from build123d import *

# Parameters (mm, degrees)
CROQUIS1_W              = 200
CROQUIS1_H              = 150
SALIENTE_EXTRUIR1_DEPTH = 3
CROQUIS2_W              = 3
CROQUIS2_H              = 150
SALIENTE_EXTRUIR2_DEPTH = 134
CROQUIS3_W              = 200
CROQUIS3_H              = 150
SALIENTE_EXTRUIR3_DEPTH = 3


with BuildPart() as part:
    # Croquis1 → Saliente-Extruir1 (new body)
    with BuildSketch(Plane(origin=(0, 0, 0), x_dir=(1, 0, 0), z_dir=(0, 1, 0))):
        with Locations((100, 75)):
            Rectangle(CROQUIS1_W, CROQUIS1_H)
    extrude(amount=SALIENTE_EXTRUIR1_DEPTH)

    # Croquis2 → Saliente-Extruir2 (add)
    with BuildSketch(Plane(origin=(0, 3, 0), x_dir=(1, 0, 0), z_dir=(0, 1, 0))):
        with Locations((1.5, 75)):
            Rectangle(CROQUIS2_W, CROQUIS2_H)
        with Locations((198.5, 75)):
            Rectangle(CROQUIS2_W, CROQUIS2_H)
    extrude(amount=SALIENTE_EXTRUIR2_DEPTH)

    # Croquis3 → Saliente-Extruir3 (add)
    with BuildSketch(Plane(origin=(0, 137, 0), x_dir=(1, 0, 0), z_dir=(0, 1, 0))):
        with Locations((100, 75)):
            Rectangle(CROQUIS3_W, CROQUIS3_H)
    extrude(amount=SALIENTE_EXTRUIR3_DEPTH)


solid = part.part
Verification items for the finished model (mm, model axes). A direction names the side the tool comes from. Coordinates: 2 decimals unless noted, no trailing zeros. Order: outer loops, then holes, each group sorted by start corner. A loop starts at its lowest first (then second) coordinate and runs counter-clockwise, first axis right, second up. Notation, with made-up numbers: (54, 89.25) -> (67, 89.25) arc R21 ccw to (67, 126.25) -> close; hole circle Ø4 at (26, -23). An arc over 180 degrees is marked (long way). Put each result on its own line as item: value. Start each with the question number.
1. Access from +Z, -Z, +X, -X, +Y, -Y to the whole of each face (thin tool, end or side, straight path). Record for faces 1 (the flat face through (99, 3, -76)), 2 (the flat face through (99, 0, -76)).
2. Material ranges on L1, parallel to Y at x = 169, z = -104; L2, parallel to X at y = 73, z = -49, recorded low to high. Write a range as [from, to].
3. Mould release check, pull along X, two halves, no side actions. Record for faces 3 (the flat face through (3, 69, -74)), 4 (the flat face through (100, 2, -150)), 5 (the flat face through (200, 69, -74)), 6 (the flat face through (0, 69, -74)): released by +X, released by -X, zero draft, split by the parting line, or undercut.
4. Cross-section at A-A, the plane y = 125. Record the boundary of the cut face in (x, z).
5. Cross-section at B-B, the plane x = 121. Record the boundary of the cut face in (y, z).
6. Cross-section at C-C, the plane z = -39. Record the boundary of the cut face in (x, y).
Computed:
1. face 1: +Z, -Z
1. face 2: +Z, -Z, +X, -X, -Y
2. L1: [0, 3], [137, 140]
2. L2: [0, 3], [197, 200]
3. face 3: undercut
3. face 4: zero draft
3. face 5: released by +X
3. face 6: released by -X
4. outline: (0, -150) -> (3, -150) -> (3, 0) -> (0, 0) -> close; (197, -150) -> (200, -150) -> (200, 0) -> (197, 0) -> close
5. outline: (0, -150) -> (3, -150) -> (3, 0) -> (0, 0) -> close; (137, -150) -> (140, -150) -> (140, 0) -> (137, 0) -> close
6. outline: (0, 0) -> (200, 0) -> (200, 140) -> (0, 140) -> close; hole (3, 3) -> (197, 3) -> (197, 137) -> (3, 137) -> close
